```python
from build123d import *

# Parameters (mm, degrees)
F0_W      = 12
F0_H      = 23
F1_DEPTH  = 22
F3_W      = 12
F3_H      = 4.5
F4_DEPTH  = 2.5
F6_DEPTH  = 18.001
F8_DEPTH  = 4.5
F9_R      = 2.425
F10_DEPTH = 3
F11_R     = 3.742917
F12_DEPTH = 25
F13_R     = 2.770584
F14_DEPTH = 220


with BuildPart() as f1:
    # F0 (on Top) → F1 (new body)
    with BuildSketch(Plane.XY):
        with Locations((6, 11.5)):
            Rectangle(F0_W, F0_H)
    extrude(amount=F1_DEPTH)

    # F3 (on offset) → F4 (join)
    with BuildSketch(Plane.XY.offset(15.5)):
        with Locations((6, 25.25)):
            Rectangle(F3_W, F3_H)
        with Locations((6, -2.25)):
            Rectangle(F3_W, F3_H)
    extrude(amount=F4_DEPTH)

    # F5 (on face) → F6 (cut, through all)
    with BuildSketch(Plane.XY.offset(18)):
        with BuildLine():
            ThreePointArc((5.425, 26.158295), (5.481589, 24.30826), (7.075, 25.25))
            ThreePointArc((7.075, 25.25), (6.94174, 25.768411), (6.575, 26.158295))
            ThreePointArc((6.575, 26.158295), (6, 26.325), (5.425, 26.158295))
        make_face()
        with BuildLine():
            ThreePointArc((5.425, 26.158295), (6, 26.325), (6.575, 26.158295))
            Line((6.575, 26.158295), (6.575, 27.5))
            Line((6.575, 27.5), (5.425, 27.5))
            Line((5.425, 27.5), (5.425, 26.158295))
        make_face()
        with BuildLine():
            Line((5.425, -4.5), (6.575, -4.5))
            Line((6.575, -4.5), (6.575, -3.158295))
            ThreePointArc((6.575, -3.158295), (6, -3.325), (5.425, -3.158295))
            Line((5.425, -3.158295), (5.425, -4.5))
        make_face()
        with BuildLine():
            ThreePointArc((5.425, -3.158295), (6, -3.325), (6.575, -3.158295))
            ThreePointArc((6.575, -3.158295), (6.94174, -2.768411), (7.075, -2.25))
            ThreePointArc((7.075, -2.25), (5.481589, -1.30826), (5.425, -3.158295))
        make_face()
    extrude(amount=-F6_DEPTH, mode=Mode.SUBTRACT)

    # F7 (on face) → F8 (join)
    with BuildSketch(Plane.XY.offset(22)):
        with BuildLine():
            ThreePointArc((8.676815, 11.630208), (11.102004, 13.84254), (12, 17))
            ThreePointArc((12, 17), (2.84254, 22.102004), (3.323185, 11.630208))
            ThreePointArc((3.323185, 11.630208), (6, 11), (8.676815, 11.630208))
        make_face()
        with BuildLine():
            ThreePointArc((8.676815, 11.630208), (6, 11), (3.323185, 11.630208))
            ThreePointArc((3.323185, 11.630208), (6, 8.25), (8.676815, 11.630208))
        make_face()
    extrude(amount=F8_DEPTH)

    # F9 (on face) → F10 (join)
    with BuildSketch(Plane.XY.offset(26.5)):
        with Locations((6, 17)):
            Circle(F9_R)
    extrude(amount=F10_DEPTH)

    # F11 (on offset) → F12 (join)
    with BuildSketch(Plane.XY.offset(15.5)):
        with Locations((5.770345, 16.935842)):
            Circle(F11_R)
    extrude(amount=F12_DEPTH)

    # F13 (on offset) → F14 (join)
    with BuildSketch(Plane.XY.offset(15.5)):
        with Locations((6.120555, 17.043775)):
            Circle(F13_R)
    extrude(amount=F14_DEPTH)


solid = f1.part
```
Design review of the part built by this model. Coordinates are the model's own, in mm. A direction names the side the tool comes from. Round coordinates to 2 decimals unless told otherwise and drop trailing zeros. Write each loop counter-clockwise with the first axis right and the second up, starting at its lowest first coordinate (ties: lowest second). Pieces come first, ordered by that corner, then holes. Notation, with made-up numbers: (-24.5, 56) -> (-17.5, 56) arc R27 cw to (-17.5, 74) -> close; hole circle Ø3 at (-38.5, 41). An arc over 180 degrees is marked (long way). Write item = value, one per line. Start each with the question number.
1) Tool access review of faces 1 (the face through (3.92, 15.36, 136.64)), 2 (the face through (6, 7, 22)), 3 (the face through (6, 23, 20)): name each direction out of +Z, -Z, +X, -X, +Y, -Y from which nothing blocks a thin tool from reaching the whole face with its end or side.
2) Mouldability with a two-part tool opening along Y and no side actions: class faces 4 (the face through (5.93, 8.25, 24.22)), 5 (the face through (1, 22, 22)), 6 (the face through (6, 23, 8)) as +Y half, -Y half, draft (parallel to the pull), parting line (faces both ways), or undercut.
3) Wall thickness on probe 1 along X at (y, z) = (25.25, 17.3) (3 decimals); probe 2 along X at (y, z) = (-2, 17); probe 3 along Z at (x, y) = (10, 5): over which ranges is each line inside the solid? List them lowest first. Write a range as from..to.
4) Take a section at A-A, the plane z = 143. State the section outline as (x, y) points, plus the area to 3 significant figures.
5) Clearance check with flat-ended pins moving along their axes: pin 1 (1.5 mm diameter, centred on y = 27, z = 17, fed in from -X); pin 2 (1.8 mm diameter, centred on x = 10, y = 19.5, fed in from +Z); pin 3 (3.5 mm diameter, centred on x = 5, y = -3, fed in from -Z); pin 4 (1.8 mm diameter, centred on x = 2, y = 19.5, fed in from +Z). State where each tip first meets the part, or that it passes through.
Results list:
q1.face_1 = +Z
q1.face_2 = +Z, -Y
q1.face_3 = +Z, +X, -X, +Y
q2.face_4 = undercut
q2.face_5 = draft
q2.face_6 = +Y half
q3.probe_1 = 0..4.925, 7.075..12
q3.probe_2 = 0..4.95, 7.05..12
q3.probe_3 = 0..22
q4.outline = circle Ø5.54 at (6.12, 17.04)
q4.area = 24.1 mm²
q5.pin_1 = 0
q5.pin_2 = 26.5
q5.pin_3 = 15.5
q5.pin_4 = 40.5
